Verification items for the finished model (mm, model axes). Face numbers are marked on the shaded views. A direction names the side the tool comes from. Round coordinates to 2 decimals unless told otherwise and drop trailing zeros. Write each loop counter-clockwise with the first axis right and the second up, starting at its lowest first coordinate (ties: lowest second). Pieces come first, ordered by that corner, then holes. Notation, with made-up numbers: (66, 59.5) - (90, 59.5) arc R16 ccw to (90, 71.5) - close; hole circle Ø3 at (11.5, -1). An arc over 180 degrees is marked (long way). Write each question's results on one line, items separated by ' | '.
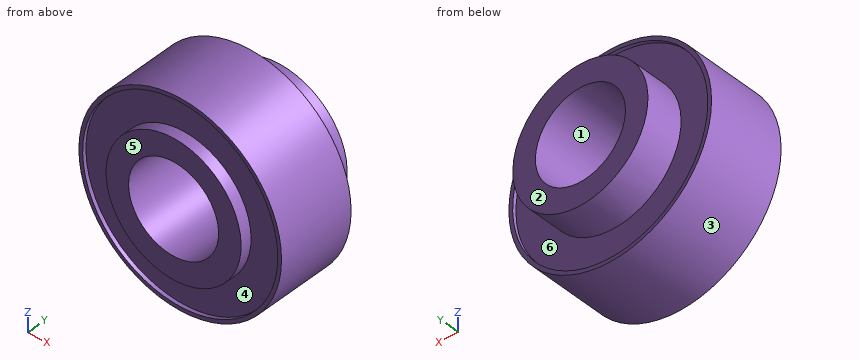
```python
from build123d import *

# Parameters (mm, degrees)
SKETCH_1_R          = 13.5
EXTRUDE_1_DEPTH     = 10.5
SKETCH_2_R          = 13
CUT_EXTRUDE_1_DEPTH = 0.5
CUT_EXTRUDE_START   = -0.5
SKETCH_3_R          = 13
CUT_EXTRUDE_2_DEPTH = 0.5
SKETCH_4_R          = 6
CUT_EXTRUDE_3_DEPTH = 22.552262062
EXTRUDE_START       = 5
SKETCH_5_R          = 9
SKETCH_5_R_2        = 6
EXTRUDE_2_DEPTH     = 5
SKETCH_6_R          = 9
SKETCH_6_R_2        = 6
EXTRUDE_3_DEPTH     = 1.5


with BuildPart() as part:
    # Эскиз1 → Бобышка-Вытянуть1 (new body)
    with BuildSketch(Plane(origin=(0, 0, 0), x_dir=(1, 0, 0), z_dir=(0, 1, 0))):
        with Locations(Location((0, 0, 0), (0, 0, 90))):
            Circle(SKETCH_1_R)
    extrude(amount=EXTRUDE_1_DEPTH)

    # Эскиз2 → Вырез-Вытянуть1 (cut)
    with BuildSketch(Plane(origin=(0, 10.5, 0), x_dir=(1, 0, 0), z_dir=(0, 1, 0))):
        with Locations(Location((0, 0, 0), (0, 0, 270))):
            Circle(SKETCH_2_R)
    extrude(amount=-CUT_EXTRUDE_1_DEPTH, mode=Mode.SUBTRACT)

    # Эскиз3 → Вырез-Вытянуть2 (cut)
    with BuildSketch(Plane.XZ.offset(CUT_EXTRUDE_START)):
        with Locations(Location((0, 0, 0), (0, 0, 90))):
            Circle(SKETCH_3_R)
    extrude(amount=CUT_EXTRUDE_2_DEPTH, mode=Mode.SUBTRACT)

    # Эскиз4 → Вырез-Вытянуть3 (cut, through all)
    with BuildSketch(Plane(origin=(0, 10, 0), x_dir=(1, 0, 0), z_dir=(0, 1, 0))):
        with Locations(Location((0, 0, 0), (0, 0, 270))):
            Circle(SKETCH_4_R)
    extrude(amount=-CUT_EXTRUDE_3_DEPTH, mode=Mode.SUBTRACT)

    # Эскиз5 → Бобышка-Вытянуть2 (add)
    with BuildSketch(Plane(origin=(0, 10, 0), x_dir=(1, 0, 0), z_dir=(0, 1, 0)).offset(EXTRUDE_START)):
        with Locations(Location((0, 0, 0), (0, 0, 270))):
            Circle(SKETCH_5_R)
        with Locations(Location((0, 0, 0), (0, 0, 270))):
            Circle(SKETCH_5_R_2, mode=Mode.SUBTRACT)
    extrude(amount=-EXTRUDE_2_DEPTH)

    # Эскиз6 → Бобышка-Вытянуть3 (add)
    with BuildSketch(Plane.XZ.offset(-0.5)):
        with Locations(Location((0, 0, 0), (0, 0, 90))):
            Circle(SKETCH_6_R)
        with Locations(Location((0, 0, 0), (0, 0, 90))):
            Circle(SKETCH_6_R_2, mode=Mode.SUBTRACT)
    extrude(amount=EXTRUDE_3_DEPTH)


solid = part.part
```
(1) Section check C-C (y = 5). Record the cut outline in (x, z), plus the area to 3 significant figures.
Answer:
outline: circle Ø27 at (0, 0); hole circle Ø12 at (0, 0) | area: 459 mm2
(2) Go/stop test with flat-tipped pins: pin 1 Ø4 at (y, z) = (9.5, -10.5) entering from -X; pin 2 Ø3 at (y, z) = (1.5, -7) entering from +X; pin 3 Ø7 at (x, z) = (0, 0) entering from -Y; pin 4 Ø5 at (x, y) = (-10.5, 8) entering from +Z. Record where each tip stops, or that it passes through.
Answer:
pin 1: x = -10.49 | pin 2: x = 12.33 | pin 3: through | pin 4: z = 10.87
(3) Set-up check for the marked faces 4, 5 and 6: record each of +Z, -Z, +X, -X, +Y, -Y from which the full face is reachable in a straight line by a thin tool's end or side.
Answer:
face 4: -Y | face 5: +Z, -Z, +X, -X, -Y | face 6: +Y
(4) Section check D-D (x = -10). Record the cut outline in (y, z), plus the area to 3 significant figures.
Answer:
outline: (0, -9.07) - (10.5, -9.07) - (10.5, -8.31) - (10, -8.31) - (10, 8.31) - (10.5, 8.31) - (10.5, 9.07) - (0, 9.07) - (0, 8.31) - (0.5, 8.31) - (0.5, -8.31) - (0, -8.31) - close | area: 174 mm2
(5) Section check B-B (z = 0). Record the cut outline in (x, y), plus the area to 4 significant figures.
Answer:
outline: (-13.5, 0) - (-13, 0) - (-13, 0.5) - (-9, 0.5) - (-9, -1) - (-6, -1) - (-6, 15) - (-9, 15) - (-9, 10) - (-13, 10) - (-13, 10.5) - (-13.5, 10.5) - close; (6, -1) - (9, -1) - (9, 0.5) - (13, 0.5) - (13, 0) - (13.5, 0) - (13.5, 10.5) - (13, 10.5) - (13, 10) - (9, 10) - (9, 15) - (6, 15) - close | area: 182.5 mm2
(6) Thickness scan on L1, parallel to X at y = 10.45, z = 0; L2, parallel to Y at x = -7, z = -9; L3, parallel to Z at x = 0.5, y = 6.5. Record the ranges inside material, lowest first.
Answer:
L1: -13.5 to -13, -9 to -6, 6 to 9, 13 to 13.5 | L2: 0.5 to 10 | L3: -13.49 to -5.98, 5.98 to 13.49
(7) Section check A-A (x = 0). Record the cut outline in (y, z), plus the area to 4 significant figures.
Answer:
outline: (-1, -9) - (0.5, -9) - (0.5, -13) - (0, -13) - (0, -13.5) - (10.5, -13.5) - (10.5, -13) - (10, -13) - (10, -9) - (15, -9) - (15, -6) - (-1, -6) - close; (-1, 6) - (15, 6) - (15, 9) - (10, 9) - (10, 13) - (10.5, 13) - (10.5, 13.5) - (0, 13.5) - (0, 13) - (0.5, 13) - (0.5, 9) - (-1, 9) - close | area: 182.5 mm2
(8) Mould release check, pull along X, two halves, no side actions. Record for the marked faces 1, 2 and 3: released by +X, released by -X, zero draft, split by the parting line, or undercut.
Answer:
face 1: undercut | face 2: zero draft | face 3: split by the parting line
